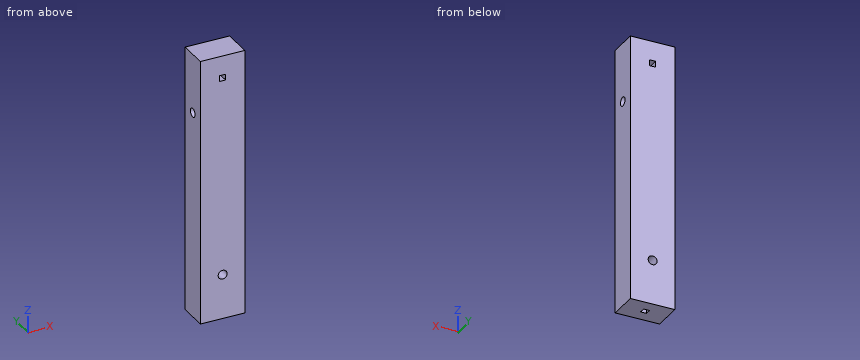
from build123d import *

# Parameters (mm, degrees)
SKETCH1_W           = 15
SKETCH1_H           = 90
BOSS_EXTRUDE1_DEPTH = 10
SKETCH2_R           = 1.5
CUT_EXTRUDE1_DEPTH  = 49.476798574
SKETCH5_W           = 2
SKETCH5_H           = 2
CUT_EXTRUDE4_DEPTH  = 47.703854231
SKETCH6_R           = 1.5
CUT_EXTRUDE5_DEPTH  = 47.703854231
SKETCH7_W           = 2
SKETCH7_H           = 2
CUT_EXTRUDE6_DEPTH  = 15


with BuildPart() as part:
    # Sketch1 → Boss-Extrude1 (new body)
    with BuildSketch(Plane(origin=(0, 0, 0), x_dir=(1, 0, 0), z_dir=(0, 1, 0))):
        Rectangle(SKETCH1_W, SKETCH1_H)
    extrude(amount=BOSS_EXTRUDE1_DEPTH)

    # Sketch2 → Cut-Extrude1 (cut, through all)
    with BuildSketch(Plane(origin=(7.5, 0, 0), x_dir=(0, 0, -1), z_dir=(1, 0, 0))):
        with Locations((-25, 5)):
            Circle(SKETCH2_R)
    extrude(amount=-CUT_EXTRUDE1_DEPTH, mode=Mode.SUBTRACT)

    # Sketch5 → Cut-Extrude4 (cut, through all)
    with BuildSketch(Plane.XZ):
        with Locations((0, 37.5)):
            Rectangle(SKETCH5_W, SKETCH5_H)
    extrude(amount=-CUT_EXTRUDE4_DEPTH, mode=Mode.SUBTRACT)

    # Sketch6 → Cut-Extrude5 (cut, through all)
    with BuildSketch(Plane(origin=(0, 10, 0), x_dir=(-1, 0, 0), z_dir=(0, 1, 0))):
        with Locations(Location((0, -30, 0), (0, 0, 90))):
            Circle(SKETCH6_R)
    extrude(amount=-CUT_EXTRUDE5_DEPTH, mode=Mode.SUBTRACT)

    # Sketch7 → Cut-Extrude6 (cut)
    with BuildSketch(Plane(origin=(0, 0, -45), x_dir=(-1, 0, 0), z_dir=(0, 0, -1))):
        with Locations((0, 5)):
            Rectangle(SKETCH7_W, SKETCH7_H)
    extrude(amount=-CUT_EXTRUDE6_DEPTH, mode=Mode.SUBTRACT)


solid = part.part
Part model, mm, in its own coordinate system. Coordinates: 2 decimals unless noted, no trailing zeros. Loops run counter-clockwise (first coordinate to the right, second up) from the corner with the lowest first, then second, coordinate; pieces in that order, holes last. Notation, with made-up numbers: M 51,60.5 L 104,60.5 A14 cw 104,81.5 Z; hole C 70.25,47 d7. An arc over 180 degrees is marked long. Use a Markdown table: item, result. Add a question column.
Q1. Pin check, flat tips, straight feed: P1, Ø0.6, axis at x = 0.5, y = 4.5, coming from the -Z side; P2, Ø1.8, axis at x = 0, z = -30, coming from the +Y side. Stop position of each tip, or through.
Q2. Cut at A-A (y = 5). Write the cut outline in (x, z).
Q3. Cut at C-C (x = 0). Write the cut outline in (y, z).
Q4. Cut at D-D (z = 25). Write the cut outline in (x, y), and give its area (3 significant figures).
Q5. Probe L1, parallel to Y at x = -0.5, z = 25; L2, parallel to X at y = 7.5, z = -30; L3, parallel to Z at x = 0.75, y = 5.25. List the from-to ranges inside material, lowest first.
Q6. Cut at B-B (z = -30). Write the cut outline in (x, y), and give its area (3 significant figures).
Worked out:
| question | item | result |
|---|---|---|
| 1 | P1 | stops at z = -28.73 |
| 1 | P2 | passes through |
| 2 | outline | M -7.5,-45 L -1,-45 L -1,-31.12 A1.5 cw long 1,-31.12 L 1,-45 L 7.5,-45 L 7.5,23.5 L -7.5,23.5 Z; M -7.5,26.5 L 7.5,26.5 L 7.5,45 L -7.5,45 Z; hole M -1,36.5 L 1,36.5 L 1,38.5 L -1,38.5 Z |
| 3 | outline | M 0,-45 L 4,-45 L 4,-31.5 L 0,-31.5 Z; M 0,-28.5 L 10,-28.5 L 10,36.5 L 0,36.5 Z; M 0,38.5 L 10,38.5 L 10,45 L 0,45 Z; M 6,-45 L 10,-45 L 10,-31.5 L 6,-31.5 Z; hole C 5,25 d3 |
| 4 | outline | M -7.5,0 L 7.5,0 L 7.5,3.5 L -7.5,3.5 Z; M -7.5,6.5 L 7.5,6.5 L 7.5,10 L -7.5,10 Z |
| 4 | area | 105 mm2 |
| 5 | L1 | y = 0 to 3.5, 6.5 to 10 |
| 5 | L2 | x = -7.5 to -1.5, 1.5 to 7.5 |
| 5 | L3 | z = -28.7 to 23.52, 26.48 to 36.5, 38.5 to 45 |
| 6 | outline | M -7.5,0 L -1.5,0 L -1.5,10 L -7.5,10 Z; M 1.5,0 L 7.5,0 L 7.5,10 L 1.5,10 Z |
| 6 | area | 120 mm2 |
